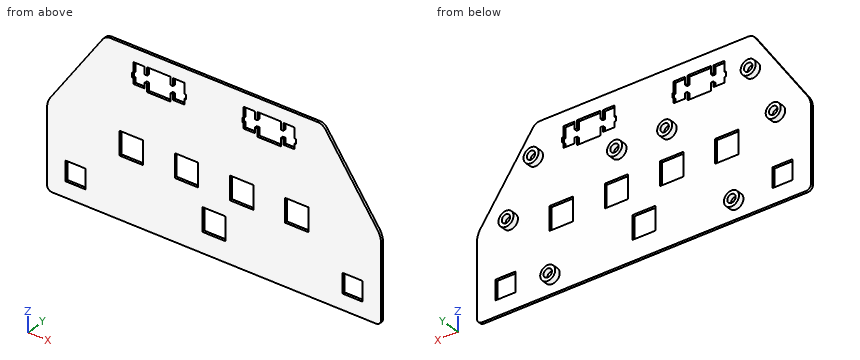
```python
from build123d import *

# Parameters (mm, degrees)
SKETCH_1_W      = 14
SKETCH_1_H      = 14
SKETCH_1_W_2    = 12
SKETCH_1_H_2    = 11.7
EXTRUDE_1_DEPTH = 1.5
SKETCH_2_R      = 4.5
SKETCH_2_R_2    = 2.5
EXTRUDE_2_DEPTH = 5
SKETCH_3_R      = 2.5
EXTRUDE_3_DEPTH = 2


with BuildPart() as part:
    # 草图1 → 凸台-拉伸1 (new body)
    with BuildSketch(Plane(origin=(0, 0, 0), x_dir=(1, 0, 0), z_dir=(0, 1, 0))):
        with BuildLine():
            Line((197, 0), (3, 0))
            ThreePointArc((3, 0), (0.878679656, -0.878679656), (0, -3))
            Line((0, -3), (0, -47))
            ThreePointArc((0, -47), (0.538734236, -49.830178992), (1.720387033, -52.457695762))
            Line((1.720387033, -52.457695762), (33.279612967, -97.542304238))
            ThreePointArc((33.279612967, -97.542304238), (35.317699373, -99.389808931), (38, -100))
            Line((38, -100), (162, -100))
            ThreePointArc((162, -100), (164.682300627, -99.389808931), (166.720387033, -97.542304238))
            Line((166.720387033, -97.542304238), (198.279612967, -52.457695762))
            ThreePointArc((198.279612967, -52.457695762), (199.461265764, -49.830178992), (200, -47))
            Line((200, -47), (200, -3))
            ThreePointArc((200, -3), (199.121320344, -0.878679656), (197, 0))
        make_face()
        with Locations((100, -19)):
            Rectangle(SKETCH_1_W, SKETCH_1_H, mode=Mode.SUBTRACT)
        with Locations((83.5, -43)):
            Rectangle(SKETCH_1_W, SKETCH_1_H, mode=Mode.SUBTRACT)
        with Locations((116.5, -43)):
            Rectangle(SKETCH_1_W, SKETCH_1_H, mode=Mode.SUBTRACT)
        with Locations((50.5, -43)):
            Rectangle(SKETCH_1_W, SKETCH_1_H, mode=Mode.SUBTRACT)
        with Locations((149.5, -43)):
            Rectangle(SKETCH_1_W, SKETCH_1_H, mode=Mode.SUBTRACT)
        Polygon((60, -78), (74, -78), (74, -82.7), (75.525, -82.7), (75.525, -79.47), (82.275, -79.47), (82.275, -82.7), (83.1, -82.7), (83.1, -85.5), (82.275, -85.5), (82.275, -91.77), (75.525, -91.77), (75.525, -87.3), (74, -87.3), (74, -92), (60, -92), (60, -87.3), (58.475, -87.3), (58.475, -91.77), (51.725, -91.77), (51.725, -85.5), (50.9, -85.5), (50.9, -82.7), (51.725, -82.7), (51.725, -79.47), (58.475, -79.47), (58.475, -82.7), (60, -82.7), align=None, mode=Mode.SUBTRACT)
        Polygon((140, -78), (126, -78), (126, -82.7), (124.475, -82.7), (124.475, -79.47), (117.725, -79.47), (117.725, -82.7), (116.9, -82.7), (116.9, -85.5), (117.725, -85.5), (117.725, -91.77), (124.475, -91.77), (124.475, -87.3), (126, -87.3), (126, -92), (140, -92), (140, -87.3), (141.525, -87.3), (141.525, -91.77), (148.275, -91.77), (148.275, -85.5), (149.1, -85.5), (149.1, -82.7), (148.275, -82.7), (148.275, -79.47), (141.525, -79.47), (141.525, -82.7), (140, -82.7), align=None, mode=Mode.SUBTRACT)
        with Locations((17, -15.1)):
            Rectangle(SKETCH_1_W_2, SKETCH_1_H_2, mode=Mode.SUBTRACT)
        with Locations((183, -15.1)):
            Rectangle(SKETCH_1_W_2, SKETCH_1_H_2, mode=Mode.SUBTRACT)
    extrude(amount=EXTRUDE_1_DEPTH)

    # 草图2 → 凸台-拉伸2 (add)
    # profile 1 of 8: a face of its own
    with BuildSketch(Plane(origin=(0, 0, 0), x_dir=(1, 0, 0), z_dir=(0, 1, 0))):
        with Locations(Location((35, -80, 0), (0, 0, 90))):
            Circle(SKETCH_2_R)
        with Locations(Location((35, -80, 0), (0, 0, 90))):
            Circle(SKETCH_2_R_2, mode=Mode.SUBTRACT)
    # profile 2 of 8: a face of its own
    with BuildSketch(Plane(origin=(0, 0, 0), x_dir=(1, 0, 0), z_dir=(0, 1, 0))):
        with Locations(Location((20, -50, 0), (0, 0, 90))):
            Circle(SKETCH_2_R)
        with Locations(Location((20, -50, 0), (0, 0, 90))):
            Circle(SKETCH_2_R_2, mode=Mode.SUBTRACT)
    # profile 3 of 8: a face of its own
    with BuildSketch(Plane(origin=(0, 0, 0), x_dir=(1, 0, 0), z_dir=(0, 1, 0))):
        with Locations(Location((45, -10, 0), (0, 0, 90))):
            Circle(SKETCH_2_R)
        with Locations(Location((45, -10, 0), (0, 0, 90))):
            Circle(SKETCH_2_R_2, mode=Mode.SUBTRACT)
    # profile 4 of 8: a face of its own
    with BuildSketch(Plane(origin=(0, 0, 0), x_dir=(1, 0, 0), z_dir=(0, 1, 0))):
        with Locations(Location((85, -65, 0), (0, 0, 90))):
            Circle(SKETCH_2_R)
        with Locations(Location((85, -65, 0), (0, 0, 90))):
            Circle(SKETCH_2_R_2, mode=Mode.SUBTRACT)
    # profile 5 of 8: a face of its own
    with BuildSketch(Plane(origin=(0, 0, 0), x_dir=(1, 0, 0), z_dir=(0, 1, 0))):
        with Locations(Location((115, -65, 0), (0, 0, 90))):
            Circle(SKETCH_2_R)
        with Locations(Location((115, -65, 0), (0, 0, 90))):
            Circle(SKETCH_2_R_2, mode=Mode.SUBTRACT)
    # profile 6 of 8: a face of its own
    with BuildSketch(Plane(origin=(0, 0, 0), x_dir=(1, 0, 0), z_dir=(0, 1, 0))):
        with Locations(Location((165, -80, 0), (0, 0, 90))):
            Circle(SKETCH_2_R)
        with Locations(Location((165, -80, 0), (0, 0, 90))):
            Circle(SKETCH_2_R_2, mode=Mode.SUBTRACT)
    # profile 7 of 8: a face of its own
    with BuildSketch(Plane(origin=(0, 0, 0), x_dir=(1, 0, 0), z_dir=(0, 1, 0))):
        with Locations(Location((155, -10, 0), (0, 0, 90))):
            Circle(SKETCH_2_R)
        with Locations(Location((155, -10, 0), (0, 0, 90))):
            Circle(SKETCH_2_R_2, mode=Mode.SUBTRACT)
    # profile 8 of 8: a face of its own
    with BuildSketch(Plane(origin=(0, 0, 0), x_dir=(1, 0, 0), z_dir=(0, 1, 0))):
        with Locations(Location((180, -50, 0), (0, 0, 90))):
            Circle(SKETCH_2_R)
        with Locations(Location((180, -50, 0), (0, 0, 90))):
            Circle(SKETCH_2_R_2, mode=Mode.SUBTRACT)
    extrude(amount=EXTRUDE_2_DEPTH)

    # 草图3 → 凸台-拉伸3 (add)
    with BuildSketch(Plane(origin=(0, 0, 0), x_dir=(1, 0, 0), z_dir=(0, 1, 0))):
        with Locations(Location((180, -50, 0), (0, 0, 270))):
            Circle(SKETCH_3_R)
        with Locations(Location((165, -80, 0), (0, 0, 270))):
            Circle(SKETCH_3_R)
        with Locations(Location((115, -65, 0), (0, 0, 270))):
            Circle(SKETCH_3_R)
        with Locations(Location((155, -10, 0), (0, 0, 270))):
            Circle(SKETCH_3_R)
        with Locations(Location((45, -10, 0), (0, 0, 270))):
            Circle(SKETCH_3_R)
        with Locations(Location((20, -50, 0), (0, 0, 270))):
            Circle(SKETCH_3_R)
        with Locations(Location((35, -80, 0), (0, 0, 270))):
            Circle(SKETCH_3_R)
        with Locations(Location((85, -65, 0), (0, 0, 270))):
            Circle(SKETCH_3_R)
    extrude(amount=EXTRUDE_3_DEPTH)


solid = part.part
```
Could you check a few things on this model? Use its own coordinates, in mm. Coordinates: 2 decimals unless noted, no trailing zeros. Write each loop counter-clockwise with the first axis right and the second up, starting at its lowest first coordinate (ties: lowest second). Pieces come first, ordered by that corner, then holes. Notation, with made-up numbers: (9, 68.25) -> (48, 68.25) arc R19 ccw to (48, 86.25) -> close; hole circle Ø11 at (9.5, -25). An arc over 180 degrees is marked (long way). Return JSON: item names as keys, results as strings.
(1) Imagine slicing it at B-B, the plane x = 135. Please give me the cut outline in (y, z), then the cut area to 3 significant figures.
Numbers:
{"outline": "(0, 0) -> (1.5, 0) -> (1.5, 78) -> (0, 78) -> close; (0, 92) -> (1.5, 92) -> (1.5, 100) -> (0, 100) -> close", "area": "129 mm2"}
(2) I need wall thicknesses on L1, parallel to X at y = 3.8, z = 65; L2, parallel to X at y = 1.3, z = 12.5; L3, parallel to Z at x = 56, y = 0.6. Which ranges of each line are inside material? Lowest first, please.
Numbers:
{"L1": "x = 80.5 to 82.5, 87.5 to 89.5, 110.5 to 112.5, 117.5 to 119.5", "L2": "x = 0 to 11, 23 to 93, 107 to 177, 189 to 200", "L3": "z = 0 to 36, 50 to 79.47, 91.77 to 100"}
(3) Imagine slicing it at C-C, the plane x = 115. Please give me the cut outline in (y, z), then the cut area to 4 significant figures.
Numbers:
{"outline": "(0, 0) -> (1.5, 0) -> (1.5, 36) -> (0, 36) -> close; (0, 50) -> (1.5, 50) -> (1.5, 60.5) -> (5, 60.5) -> (5, 62.5) -> (2, 62.5) -> (2, 67.5) -> (5, 67.5) -> (5, 69.5) -> (1.5, 69.5) -> (1.5, 100) -> (0, 100) -> close", "area": "145.5 mm2"}
(4) I'm going to push flat-ended pins straight in: pin 1 (0.8 mm diameter, centred on y = 0.5, z = 89.5, fed in from -X); pin 2 (0.8 mm diameter, centred on y = 0.5, z = 81, fed in from -X); pin 3 (1.5 mm diameter, centred on x = 53.5, z = 71, fed in from +Y). Where does each tip first touch, or does it pass through?
Numbers:
{"pin 1": "stops at x = 27.37", "pin 2": "stops at x = 21.42", "pin 3": "stops at y = 1.5"}
(5) Imagine slicing it at D-D, the plane x = 20. Please give me the cut outline in (y, z), then the cut area to 3 significant figures.
Numbers:
{"outline": "(0, 0) -> (1.5, 0) -> (1.5, 9.25) -> (0, 9.25) -> close; (0, 20.95) -> (1.5, 20.95) -> (1.5, 45.5) -> (5, 45.5) -> (5, 47.5) -> (2, 47.5) -> (2, 52.5) -> (5, 52.5) -> (5, 54.5) -> (1.5, 54.5) -> (1.5, 78.57) -> (0, 78.57) -> close", "area": "117 mm2"}
(6) Imagine slicing it at A-A, the plane y = 2.9. Count the separate pieces of the cut face and the enclosed holes in it, then the cut area to 3 significant figures.
Numbers:
{"separate pieces": "8", "enclosed holes": "8", "area": "352 mm2"}
